```python
from build123d import *

# Parameters (mm, degrees)
EXTRUDE_THIN1_DEPTH   = 38.1
SKETCH2_R             = 6.3627
CUT_EXTRUDE1_DEPTH    = 68.873747686
F_2_CLEARANCE_HOLE1_D = 2.4384


with BuildPart() as part:
    # Sketch1 → Extrude-Thin1 (new body)
    with BuildSketch(Plane(origin=(0, 0, 0), x_dir=(1, 0, 0), z_dir=(0, 1, 0))):
        Polygon((0, 38.1), (0, 0), (38.1, 0), (38.1, -3.175), (-3.175, -3.175), (-3.175, 38.1), align=None)
    extrude(amount=EXTRUDE_THIN1_DEPTH)

    # Sketch2 → Cut-Extrude1 (cut, through all)
    with BuildSketch(Plane.ZY.offset(3.175)):
        with Locations((-17.4625, 19.05)):
            Circle(SKETCH2_R)
    extrude(amount=-CUT_EXTRUDE1_DEPTH, mode=Mode.SUBTRACT)

    # #2 Clearance Hole1 (through all)
    with Locations(Plane.ZY.offset(3.175)):
        with Locations((-27.0862073, 13.49375), (-17.4625, 30.1625), (-7.8387927, 13.49375)):
            Hole(F_2_CLEARANCE_HOLE1_D / 2)


solid = part.part
```
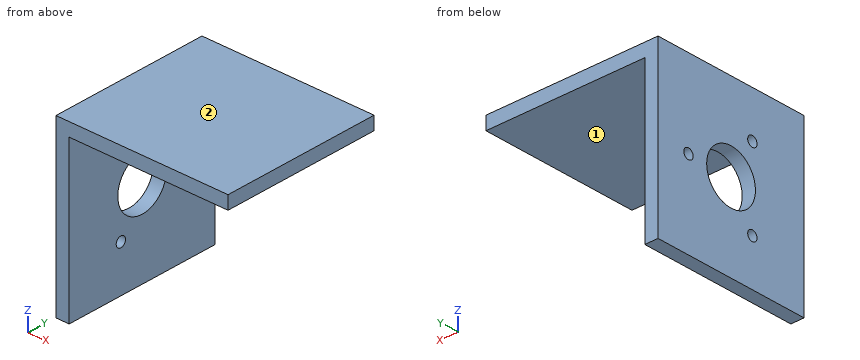
Geometry check sheet. Reference: the model listing, model coordinates, mm. Face numbers are marked on the shaded views. A direction names the side the tool comes from. Round coordinates to 2 decimals unless told otherwise and drop trailing zeros. Order: outer loops, then holes, each group sorted by start corner. A loop starts at its lowest first (then second) coordinate and runs counter-clockwise, first axis right, second up. Notation, with made-up numbers: (-14, -38.75) -> (-10, -38.75) arc R16 ccw to (-10, -18.75) -> close; hole circle Ø4 at (73.5, 60). An arc over 180 degrees is marked (long way). Return JSON: item names as keys, results as strings. Group by question number.
Q1. Tool access check on the marked faces 1 and 2. Record the directions out of +Z, -Z, +X, -X, +Y, -Y that give a thin tool (end or side, any length) a straight path to the whole face; none if there is none.
Q2. Material ranges on probe 1 along X at (y, z) = (3.5, -26.5) (3 decimals); probe 2 along Z at (x, y) = (26.5, 4) (3 decimals); probe 3 along Z at (x, y) = (-1, 18) (3 decimals), recorded low to high. Write a range as from..to.
Q3. Section check D-D, the plane x = 4. Record the boundary of the cut face in (y, z) (3 decimals), plus the area to 3 significant figures.
Q4. Section check A-A, the plane y = 19.05. Record the boundary of the cut face in (x, z) (3 decimals), plus the area to 3 significant figures.
Q5. Gauge pin test, flat ends, axial feed: pin 1 (4 mm diameter, centred on x = 22, y = 22.5, fed in from -Z); pin 2 (3 mm diameter, centred on y = 30, z = -14, fed in from +X). Record the tip position at first contact, or that the pin passes through.
Q6. Section check B-B, the plane z = -26.5. Record the boundary of the cut face in (x, y) (3 decimals).
Q7. Section check C-C, the plane y = 9. Record the boundary of the cut face in (x, z) (3 decimals).
Numbers:
{
 "1": {"face 1": "-Z, +X, +Y, -Y", "face 2": "+Z, +X, -X, +Y, -Y"},
 "2": {"probe 1": "-3.175..0", "probe 2": "0..3.175", "probe 3": "-38.1..-23.738, -11.187..3.175"},
 "3": {"outline": "(0, 0) -> (38.1, 0) -> (38.1, 3.175) -> (0, 3.175) -> close", "area": "121 mm^2"},
 "4": {"outline": "(-3.175, -38.1) -> (0, -38.1) -> (0, -23.825) -> (-3.175, -23.825) -> close; (-3.175, -11.1) -> (0, -11.1) -> (0, 0) -> (38.1, 0) -> (38.1, 3.175) -> (-3.175, 3.175) -> close", "area": "212 mm^2"},
 "5": {"pin 1": "z = 0", "pin 2": "x = 0"},
 "6": {"outline": "(-3.175, 0) -> (0, 0) -> (0, 12.425) -> (-3.175, 12.425) -> close; (-3.175, 14.563) -> (0, 14.563) -> (0, 38.1) -> (-3.175, 38.1) -> close"},
 "7": {"outline": "(-3.175, -38.1) -> (0, -38.1) -> (0, 0) -> (38.1, 0) -> (38.1, 3.175) -> (-3.175, 3.175) -> close"}
}
